The listing builds one solid part. Answer for the finished solid, in the listing's coordinates (mm). Face numbers are marked on the shaded views. A direction names the side the tool comes from. Give positions to 0.01 mm unless a question says otherwise; leave off trailing zeros. Order: outer loops, then holes, each group sorted by start corner. A loop starts at its lowest first (then second) coordinate and runs counter-clockwise, first axis right, second up. Notation, with made-up numbers: (76, -8.5) - (99, -8.5) arc R17 ccw to (99, 7.5) - close; hole circle Ø3 at (-18.75, 30.5). An arc over 180 degrees is marked (long way). Use a Markdown table: item, result. Add a question column.
1) Straight lines are drawn through the part: line 1 (Z direction, x = 22.25, y = -15.5); line 2 (Y direction, x = 36.5, z = 46.5); line 3 (Z direction, x = 40, y = -29). For each, find the intervals that lie inside material, in ascending order.
2) Find section C-C, the plane y = -45. Determine the outline of the cut face in (x, z).
3) Find section A-A, the plane y = -37. Determine the outline of the cut face in (x, z), plus the area to 3 significant figures.
4) Find section D-D, the plane z = 21. Determine the outline of the cut face in (x, y).
5) The mould has two halves that part along X. Classify the marked faces 1, 2 and 3: released by +X, released by -X, zero draft, split by the parting line, or undercut.
6) For the marked faces 4 and 5, determine the directions among +Z, -Z, +X, -X, +Y, -Y from which every point of the face is accessible in a straight line to the end or side of a thin tool.
7) Find section B-B, the plane x = 25.75. Determine the outline of the cut face in (y, z).
8) Flat-ended cylindrical pins translate along their axes: pin 1 (5 mm diameter, centred on y = -37, z = 35.5, fed in from +X); pin 2 (3.5 mm diameter, centred on x = 42, y = -5, fed in from -Z); pin 3 (8 mm diameter, centred on x = 43, y = -39, fed in from -Z); pin 4 (1.5 mm diameter, centred on x = 41, y = -19.5, fed in from +Z). Find the tip coordinate at first contact, or state that the pin passes through.
from build123d import *

# Parameters (mm, degrees)
F0_W     = 50.8
F0_H     = 50.799992591
F1_DEPTH = 50.8
F5_DEPTH = 50.8
F6_W     = 35.56
F6_H     = 10.16
F7_DEPTH = 50.8
F8_W     = 13.97
F8_H     = 10.16
F9_DEPTH = 50.8


with BuildPart() as f1:
    # F0 (on Front) → F1 (new body)
    with BuildSketch(Plane.XZ):
        with Locations((25.4, 25.3999962955)):
            Rectangle(F0_W, F0_H)
    extrude(amount=F1_DEPTH)

    # F4 (on face) → F5 (cut)
    with BuildSketch(Plane.XZ.offset(50.8)):
        Polygon((20.32, 50.799992591), (0, 50.799992591), (0, 0), (13.762652874, 0), (20.32, 0), align=None)
        with BuildLine():
            ThreePointArc((24.0402308716, 2.7991833631), (46.1192378047, 25.7211648984), (23.4431624413, 48.0526536703))
            Line((23.4431624413, 48.0526536703), (24.0402308716, 2.7991833631))
        make_face()
        with BuildLine():
            Line((50.8, 50.799992591), (27.7604617432, 50.799992591))
            ThreePointArc((27.7604617432, 50.799992591), (49.7112248054, 25.3999962955), (27.7604617432, 0))
            Line((27.7604617432, 0), (50.8, 0))
            Line((50.8, 0), (50.8, 50.799992591))
        make_face()
    extrude(amount=-F5_DEPTH, mode=Mode.SUBTRACT)

    # F6 (on offset) → F7 (cut)
    with BuildSketch(Plane.YZ.offset(50.8)):
        with Locations((-17.78, 35.56)):
            Rectangle(F6_W, F6_H)
        with Locations((-33.02, 15.24)):
            Rectangle(F6_W, F6_H)
    extrude(amount=-F7_DEPTH, mode=Mode.SUBTRACT)

    # F8 (on offset) → F9 (cut)
    with BuildSketch(Plane.XY.offset(50.8)):
        with Locations((42.6789473106, -15.24)):
            Rectangle(F8_W, F8_H)
        with Locations((27.4389473106, -35.56)):
            Rectangle(F8_W, F8_H)
    extrude(amount=-F9_DEPTH, mode=Mode.SUBTRACT)


solid = f1.part
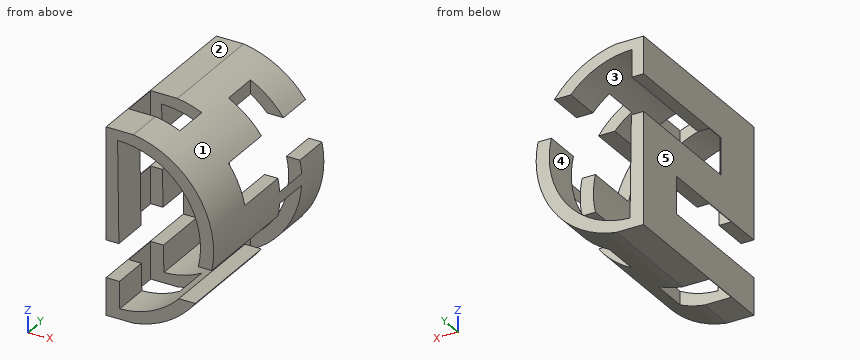
The answers:
| question | item | result |
|---|---|---|
| 1 | line 1 | 0 to 10.16, 20.32 to 30.48, 40.64 to 50.8 |
| 1 | line 2 | -50.8 to -20.32, -10.16 to 0 |
| 1 | line 3 | 5.29 to 9.94, 40.9 to 45.51 |
| 2 | outline | (20.32, 0) - (27.76, 0) arc R25.67 ccw to (44.7, 10.16) - (40.2, 10.16) arc R22.63 cw to (24.04, 2.8) - (23.94, 10.16) - (20.32, 10.16) - close; (20.32, 20.32) - (23.81, 20.32) - (23.44, 48.05) arc R22.63 cw to (45.54, 20.32) - (49.2, 20.32) arc R25.67 ccw to (27.76, 50.8) - (20.32, 50.8) - close |
| 3 | outline | (20.32, 0) - (20.45, 0) - (20.45, 10.16) - (20.32, 10.16) - close; (20.32, 20.32) - (20.45, 20.32) - (20.45, 50.8) - (20.32, 50.8) - close; (34.42, 1.92) arc R25.67 ccw to (44.7, 10.16) - (40.2, 10.16) arc R22.63 cw to (34.42, 5.61) - close; (34.42, 45.24) arc R22.63 cw to (45.54, 20.32) - (49.2, 20.32) arc R25.67 ccw to (34.42, 48.88) - close |
| 3 | area | 152 mm2 |
| 4 | outline | (20.32, -50.8) - (23.8, -50.8) - (23.8, -40.64) - (20.45, -40.64) - (20.45, -30.48) - (23.8, -30.48) - (23.8, 0) - (20.32, 0) - close; (45.68, -50.8) - (49.33, -50.8) - (49.33, -20.32) - (45.68, -20.32) - close; (45.68, -10.16) - (49.33, -10.16) - (49.33, 0) - (45.68, 0) - close |
| 5 | face 1 | released by +X |
| 5 | face 2 | zero draft |
| 5 | face 3 | undercut |
| 6 | face 4 | +Y, -Y |
| 6 | face 5 | +Z, -Z, -X, +Y, -Y |
| 7 | outline | (-50.8, 0) - (-40.64, 0) - (-40.64, 2.91) - (-50.8, 2.91) - close; (-50.8, 47.94) - (-40.64, 47.94) - (-40.64, 50.8) - (-50.8, 50.8) - close; (-30.48, 0) - (0, 0) - (0, 2.91) - (-30.48, 2.91) - close; (-30.48, 47.94) - (0, 47.94) - (0, 50.8) - (-30.48, 50.8) - close |
| 8 | pin 1 | x = 48.56 |
| 8 | pin 2 | z = 5.49 |
| 8 | pin 3 | z = 4.54 |
| 8 | pin 4 | through |
